Autodesk Inventor part; units mm, degrees
ref_plane "YZ Plane" through (0, 0, 0) normal (1, 0, 0) x (0, 1, 0)
ref_plane "XZ Plane" through (0, 0, 0) normal (0, 1, 0) x (-1, 0, 0)
ref_plane "XY Plane" through (0, 0, 0) normal (0, 0, 1) x (1, 0, 0)
sketch "スケッチ1" plane through (0, 0, 0) normal (0, 0, 1) x (1, 0, 0)
  arc A0 (3.7417, 1.55) -> (3.7417, -1.55) centre (0, 0) ccw
  circle A1 centre (-15.5, 0) radius 1.6
  circle A2 centre (-7.75, 13.4234) radius 1.6
  circle A3 centre (-7.75, -13.4234) radius 1.6
  line L0 (-7.75, 13.4234) -> (0, 0) construction
  line L1 (0, 0) -> (-7.75, -13.4234) construction
  line L2 (-15.5, 0) -> (0, 0) construction
  arc A4 (-6.3339, 18.9706) -> (-13.2621, 14.9706) centre (0, 0) ccw
  arc A5 (-19.5959, 4) -> (-19.5959, -4) centre (0, 0) ccw
  arc A6 (-13.2621, -14.9706) -> (-6.3339, -18.9706) centre (0, 0) ccw
  arc A7 (-19.5959, 4) -> (-13.2621, 14.9706) centre (-23.1306, 13.3545) ccw
  line L3 (-6.3339, 18.9706) -> (-7.75, 13.4234) construction
  line L4 (-13.2621, 14.9706) -> (-7.75, 13.4234) construction
  line L5 (-13.2621, 14.9706) -> (-6.3339, 18.9706) construction
  line L6 (-19.5959, 4) -> (-15.5, 0) construction
  line L7 (-15.5, 0) -> (-19.5959, -4) construction
  line L8 (-19.5959, -4) -> (-19.5959, 4) construction
  line L9 (-13.2621, -14.9706) -> (-6.3339, -18.9706) construction
  line L10 (-6.3339, -18.9706) -> (-7.75, -13.4234) construction
  line L11 (-7.75, -13.4234) -> (-13.2621, -14.9706) construction
  arc A8 (-13.2621, -14.9706) -> (-19.5959, -4) centre (-23.1306, -13.3545) ccw
  line L12 (8, 5.55) -> (12.3462, 5.55)
  line L13 (18, 5.55) -> (18, 1.55)
  line L14 (18, 1.55) -> (3.7417, 1.55)
  line L15 (3.7417, -1.55) -> (18, -1.55)
  line L16 (18, -1.55) -> (18, -5.55)
  line L17 (18, -5.55) -> (13.6538, -5.55)
  line L18 (-6.3339, 18.9706) -> (3, 18.9706)
  line L19 (3, 18.9706) -> (8, 5.55)
  line L20 (-6.3339, -18.9706) -> (3, -18.9706)
  line L21 (3, -18.9706) -> (8, -5.55)
  arc A9 (12.3462, 5.55) -> (13.6538, 5.55) centre (13, 6.9) ccw
  arc A10 (13.6538, -5.55) -> (12.3462, -5.55) centre (13, -6.9) ccw
  arc A11 (13.6538, 5.55) -> (12.3462, 5.55) centre (13, 6.9) ccw construction
  arc A12 (12.3462, -5.55) -> (13.6538, -5.55) centre (13, -6.9) ccw construction
  line L22 (13.6538, 5.55) -> (18, 5.55)
  line L23 (12.3462, 5.55) -> (13.6538, 5.55) construction
  line L24 (13.6538, -5.55) -> (12.3462, -5.55) construction
  line L25 (12.3462, -5.55) -> (8, -5.55)
  dimension "d18" = 8.1
  dimension "d24" = 3.2
  dimension "d25" = 3.2
  dimension "d26" = 60
  dimension "d27" = 60
  dimension "d28" = 15.5
  dimension "d29" = 3.2
  dimension "d30" = 20
  dimension "d31" = 20
  dimension "d36" = 3.1
  dimension "d37" = 1.55
  dimension "d38" = 4
  dimension "d39" = 4
  dimension "d40" = 10
  dimension "d44" = 18
  dimension "d45" = 18
  dimension "d47" = 3
  dimension "d48" = 1.35
  dimension "d49" = 3
  dimension "d50" = 1.35
  dimension "d51" = 5
  dimension "d59" = 10
  dimension "d60" = 10
  dimension "d61" = 8
  dimension "d62" = 8
  dimension "d63" = 8
  dimension "d64" = 5
extrude "押し出し1" add sketch "スケッチ1" along normal blind 6
sketch "スケッチ2" plane through (13.6538, 5.55, 0) normal (0, 1, 0) x (1, 0, 0)
  circle A0 centre (-0.6538, -3) radius 1.6
  line L0 (0, 0) -> (-1.3077, 0)
  point P0 (-13.6538, 0)
  point P1 (-0.6538, 0)
  dimension "d54" = 3.2
  dimension "d55" = 3
extrude "押し出し2" cut sketch "スケッチ2" against normal through all
fillet "フィレット1" radius 2 10 edges at (8, 5.55, 3) (3, 18.9706, 3) (-6.3339, 18.9706, 3) (-13.2621, 14.9706, 3) (-19.5959, 4, 3) (-19.5959, -4, 3) (-13.2621, -14.9706, 3) (-6.3339, -18.9706, 3) (3, -18.9706, 3) (8, -5.55, 3)
properties part number "オムニ固定する" material "アルミニウム 6061"
Check sheet for the modelled part. Datum: model origin and axes. Units: mm. A direction names the side the tool comes from. Round coordinates to 2 decimals unless told otherwise and drop trailing zeros. Loops run counter-clockwise (first coordinate to the right, second up) from the corner with the lowest first, then second, coordinate; pieces in that order, holes last. Notation, with made-up numbers: M 35,-9 L 67,-9 A27 cw 67,27 Z; hole C 76,57.5 d11. An arc over 180 degrees is marked long. Answer as a JSON object with one key per item and string values.
1. Section check A-A (x = 0). Record the boundary of the cut face in (y, z), plus the area to 3 significant figures.
Reply:
{"outline": "M -18.97,0 L -4.05,0 L -4.05,6 L -18.97,6 Z; M 4.05,0 L 18.97,0 L 18.97,6 L 4.05,6 Z", "area": "179 mm²"}
2. Section check C-C (x = 13). Record the boundary of the cut face in (y, z).
Reply:
{"outline": "M -5.4,0 L -1.55,0 L -1.55,1.4 L -5.4,1.4 Z; M -5.4,4.6 L -1.55,4.6 L -1.55,6 L -5.4,6 Z; M 1.55,0 L 5.4,0 L 5.4,1.4 L 1.55,1.4 Z; M 1.55,4.6 L 5.4,4.6 L 5.4,6 L 1.55,6 Z"}
3. Mould release check, pull along X, two halves, no side actions. Record for faces 4 (the cylindrical face through (-9.7, 17.49, 2.96)), 5 (the flat face through (11, -5.55, 3)), 6 (the cylindrical face through (-4.047, -0.156, 2.958)), 7 (the cylindrical face through (13, 5.4, 0.8)): pulls with the +X half, pulls with the -X half, needs draft (parallel to the pull), parting line crosses it, or undercut.
Reply:
{"face 4": "pulls with the -X half", "face 5": "needs draft", "face 6": "undercut", "face 7": "undercut"}
4. Gauge pin test, flat ends, axial feed: P1, Ø13, axis at x = 0, y = 0, coming from the -Z side; P2, Ø3.5, axis at x = 16, z = 2.5, coming from the +Y side; P3, Ø3.5, axis at x = 13, z = 3, coming from the -Y side; P4, Ø2.5, axis at x = 10.5, z = 3.5, coming from the -Y side. Record the tip position at first contact, or that the pin passes through.
Reply:
{"P1": "stops at z = 0", "P2": "stops at y = 5.55", "P3": "stops at y = -5.55", "P4": "stops at y = -5.55"}
5. Section check B-B (y = 0). Record the boundary of the cut face in (x, z), plus the area to 3 significant figures.
Reply:
{"outline": "M -20,0 L -17.1,0 L -17.1,6 L -20,6 Z; M -13.9,0 L -4.05,0 L -4.05,6 L -13.9,6 Z", "area": "76.5 mm²"}
6. Access from +Z, -Z, +X, -X, +Y, -Y to the whole of each face (thin tool, end or side, straight path). Record for faces 1 (the flat face through (11, 5.55, 3)), 2 (the cylindrical face through (-7.96, -15.01, 2.96)), 3 (the flat face through (11, -1.55, 3)).
Reply:
{"face 1": "+Z, -Z, +X, +Y", "face 2": "+Z, -Z", "face 3": "+Z, -Z, +X"}
7. Section check D-D (x = -7.75). Record the boundary of the cut face in (y, z).
Reply:
{"outline": "M -18.44,0 L -15.02,0 L -15.02,6 L -18.44,6 Z; M -11.82,0 L 11.82,0 L 11.82,6 L -11.82,6 Z; M 15.02,0 L 18.44,0 L 18.44,6 L 15.02,6 Z"}
8. Scan lines: line 1 (Z direction, x = 13, y = -3.25); line 2 (Y direction, x = -7.75, z = 3.2); line 3 (Y direction, x = 10, z = 1). Record each from-to range of solid material in increasing order.
Reply:
{"line 1": "z = 0 to 1.4, 4.6 to 6", "line 2": "y = -18.44 to -15.02, -11.82 to 11.82, 15.02 to 18.44", "line 3": "y = -5.55 to -1.55, 1.55 to 5.55"}
